Autodesk Inventor part; units mm, degrees
ref_plane "YZ Plane" through (0, 0, 0) normal (1, 0, 0) x (0, 1, 0)
ref_plane "XZ Plane" through (0, 0, 0) normal (0, 1, 0) x (-1, 0, 0)
ref_plane "XY Plane" through (0, 0, 0) normal (0, 0, 1) x (1, 0, 0)
sketch "Sketch1" plane through (0, 0, 0) normal (0, 0, 1) x (1, 0, 0)
  circle A0 centre (-641.35, -11.938) radius 2.667
  line L0 (-635, -25.4) -> (-787.4, -25.4)
  line L1 (-611.5558, 111.1309) -> (-611.5558, 92.0809)
  line L2 (-611.5558, 88.9059) -> (-611.5558, 92.0809)
  line L3 (-655.7192, 0) -> (-787.4, 0)
  line L4 (-611.5558, 92.0809) -> (-635, -25.4)
  line L5 (-633.655, 111.1309) -> (-660.9008, -25.4)
  line L6 (-655.8321, 0) -> (-787.4, 0)
  line L7 (-633.655, 111.1309) -> (-607.7542, 111.1309)
  line L8 (-607.7542, 111.1309) -> (-611.5558, 92.0809)
  line L9 (-660.9008, -25.4) -> (-635, -25.4)
  point P0 (0, 0)
  dimension "d1" = 25.4
extrude "Extrusion1" add sketch "Sketch1" along normal blind 3.175
properties part number "2018 Cube Backstop Mount Angle"
The model under review builds one solid part; all positions refer to its coordinate system, in mm. Round coordinates to 2 decimals unless told otherwise and drop trailing zeros. Order: outer loops, then holes, each group sorted by start corner. A loop starts at its lowest first (then second) coordinate and runs counter-clockwise, first axis right, second up. Notation, with made-up numbers: (-21.75, -6.5) -> (-10.75, -6.5) arc R19 ccw to (-10.75, 11.5) -> close; hole circle Ø3 at (85.25, 27.25). An arc over 180 degrees is marked (long way). Use CSV: the item, a comma, the result in double quotes. Start each with the question number.
(1) Consider section A-A on x = -641. Write out the cut boundary in (y, z) (3 decimals), and give its area (3 significant figures).
(2) Insertion check: pin 1 (1.5 mm diameter, centred on y = 92, z = 3, fed in from -X). The pin has a flat end and moves straight along its axis. Give the tip position at first contact, or say it passes through.
(3) Mouldability with a two-part tool opening along Y and no side actions: class faces 1 (the face through (-635, 44, 0)), 2 (the face through (-644.014, -12.055, 1.565)), 3 (the face through (-647.087, 43.821, 1.565)) as pulls with the +Y half, pulls with the -Y half, needs draft (parallel to the pull), parting line crosses it, or undercut.
(4) Consider section C-C on y = 0. Write out the cut boundary in (x, z) (3 decimals), and give its area (3 significant figures).
(5) Consider section D-D on x = -648. Write out the cut boundary in (y, z) (3 decimals).
(6) Wall thickness on probe 1 along X at (y, z) = (43.5, 1.15); probe 2 along X at (y, z) = (97, 1.7): over which ranges is each line inside the solid? List them lowest first. Write a range as from..to.
(7) Consider section B-B on z = 2.5. Write out the cut boundary in (x, y) (3 decimals), and give its area (3 significant figures).
Responses:
1,outline,"(-25.4, 0) -> (-14.582, 0) -> (-14.582, 3.175) -> (-25.4, 3.175) -> close; (-9.294, 0) -> (74.325, 0) -> (74.325, 3.175) -> (-9.294, 3.175) -> close"
1,area,"300 mm²"
2,pin 1,"x = -637.62"
3,face 1,"needs draft"
3,face 2,"undercut"
3,face 3,"pulls with the +Y half"
4,outline,"(-655.832, 0) -> (-629.931, 0) -> (-629.931, 3.175) -> (-655.832, 3.175) -> close"
4,area,"82.2 mm²"
5,outline,"(-25.4, 0) -> (39.247, 0) -> (39.247, 3.175) -> (-25.4, 3.175) -> close"
6,probe 1,"-647.15..-621.25"
6,probe 2,"-636.47..-610.57"
7,outline,"(-660.901, -25.4) -> (-635, -25.4) -> (-611.556, 92.081) -> (-607.754, 111.131) -> (-633.655, 111.131) -> close; hole circle Ø5.334 at (-641.35, -11.938)"
7,area,"3,510 mm²"
